```python
from build123d import *

# Parameters (mm, degrees)
SKETCH1_W                 = 22.5
SKETCH1_H                 = 40
BOSS_EXTRUDE1_DEPTH       = 40
SKETCH2_W                 = 5
SKETCH2_H                 = 10
CUT_EXTRUDE1_DEPTH        = 40
M3X0_5_TAPPED_HOLE2_D     = 2.5
M3X0_5_TAPPED_HOLE2_DEPTH = 6.5
M3X0_5_TAPPED_HOLE2_TIP   = 0.751075774
M3X0_5_TAPPED_HOLE3_D     = 2.5
M3X0_5_TAPPED_HOLE3_DEPTH = 6.5
M3X0_5_TAPPED_HOLE3_TIP   = 0.751075774


with BuildPart() as part:
    # Sketch1 → Boss-Extrude1 (new body)
    with BuildSketch(Plane(origin=(0, 3, 0), x_dir=(-1, 0, 0), z_dir=(0, 1, 0))):
        with Locations((5.393225555, 5.12970783)):
            Rectangle(SKETCH1_W, SKETCH1_H)
    extrude(amount=BOSS_EXTRUDE1_DEPTH)

    # Sketch2 → Cut-Extrude1 (cut)
    with BuildSketch(Plane.XY.offset(25.12970783)):
        with Locations((-14.143225555, 8)):
            Rectangle(SKETCH2_W, SKETCH2_H)
    extrude(amount=-CUT_EXTRUDE1_DEPTH, mode=Mode.SUBTRACT)

    # M3x0.5 Tapped Hole2
    with Locations(Plane.ZY.offset(16.643225555)):
        with Locations((5.12970783, 23), (5.12970783, 33)):
            Hole(M3X0_5_TAPPED_HOLE2_D / 2, depth=M3X0_5_TAPPED_HOLE2_DEPTH)
            with Locations((0, 0, -(M3X0_5_TAPPED_HOLE2_DEPTH + M3X0_5_TAPPED_HOLE2_TIP / 2))):  # 118° drill point
                Cone(0, M3X0_5_TAPPED_HOLE2_D / 2, M3X0_5_TAPPED_HOLE2_TIP, mode=Mode.SUBTRACT)

    # M3x0.5 Tapped Hole3
    with Locations(Plane.XZ.offset(-3)):
        with Locations((-2.143225555, 17.12970783), (-2.143225555, -6.87029217)):
            Hole(M3X0_5_TAPPED_HOLE3_D / 2, depth=M3X0_5_TAPPED_HOLE3_DEPTH)
            with Locations((0, 0, -(M3X0_5_TAPPED_HOLE3_DEPTH + M3X0_5_TAPPED_HOLE3_TIP / 2))):  # 118° drill point
                Cone(0, M3X0_5_TAPPED_HOLE3_D / 2, M3X0_5_TAPPED_HOLE3_TIP, mode=Mode.SUBTRACT)


solid = part.part
```
Model file for the job. Use its own axes, mm. A direction names the side the tool comes from. Give positions to 0.01 mm unless a question says otherwise; leave off trailing zeros. Write each loop counter-clockwise with the first axis right and the second up, starting at its lowest first coordinate (ties: lowest second). Pieces come first, ordered by that corner, then holes. Notation, with made-up numbers: (7, -4.5) - (60, -4.5) arc R12 cw to (60, 18.5) - close; hole circle Ø6 at (85, 45). An arc over 180 degrees is marked (long way). One line per question, with ' | ' between items. Start each with the question number.
(1) 3-axis set-ups, long thin cutter, end or side, ignore diameter. For faces 5 (the face through (-13.348, 32.521, 3.975)), 6 (the face through (-14, 13, 5)), 7 (the face through (-3, 3, 5)), 8 (the face through (-1.87, 6.3, 15.91)): which of +Z, -Z, +X, -X, +Y, -Y reach the whole face in a straight line?
(2) Slice it at A-A on x = -14. Write the cut outline in (y, z), plus the area to 3 significant figures.
(3) Two-plate mould, pull along Z, no slides. Class faces 1 (the face through (-5, 43, 5)), 2 (the face through (-13.35, 21.78, 5.4)), 3 (the face through (-5, 23, 25.13)), 4 (the face through (-1.98, 6.3, -5.63)): +Z half, -Z half, draft (parallel to the pull), parting line (faces both ways), or undercut.
(4) Wall check: line 1 along Z through (x, y) = (-13.25, 33); line 2 along X through (y, z) = (11, 9.5); line 3 along Y through (x, z) = (-15, -1.5). Give the ranges that are in metal, low to high. Write a range as from..to.
(5) Pin check, flat tips, straight feed: P1, Ø3, axis at x = -2.14, z = 17.13, coming from the -Y side; P2, Ø4, axis at x = -14.5, z = 9.5, coming from the -Y side; P3, Ø8, axis at y = 8.5, z = 2.5, coming from the -X side. Stop position of each tip, or through.
(6) Slice it at B-B on z = -12. Write the cut outline in (x, y), plus the area to 3 significant figures.
Results below:
1) face 5: -X | face 6: +Z, -Z, -X, -Y | face 7: +Z, -Z, +X, -X, -Y | face 8: -Y
2) outline: (13, -14.87) - (43, -14.87) - (43, 25.13) - (13, 25.13) - close; hole circle Ø2.5 at (23, 5.13); hole circle Ø2.5 at (33, 5.13) | area: 1,190 mm^2
3) face 1: draft | face 2: undercut | face 3: +Z half | face 4: undercut
4) line 1: -14.87..3.88, 6.38..25.13 | line 2: -11.64..5.86 | line 3: 13..43
5) P1: y = 3 | P2: y = 13 | P3: x = -11.64
6) outline: (-16.64, 13) - (-11.64, 13) - (-11.64, 3) - (5.86, 3) - (5.86, 43) - (-16.64, 43) - close | area: 850 mm^2
